from build123d import *

# Parameters (mm, degrees)
BOSS_EXTRU_1_DEPTH      = 320
ENL_V_MAT_EXTRU_1_DEPTH = 70
ESQUISSE3_R             = 150
BOSS_EXTRU_2_DEPTH      = 10
ESQUISSE4_R             = 1
ENL_V_MAT_EXTRU_2_DEPTH = 10


with BuildPart() as part:
    # Esquisse1 → Boss.-Extru.1 (new body)
    with BuildSketch(Plane(origin=(0, 0, 0), x_dir=(1, 0, 0), z_dir=(0, 1, 0))):
        with BuildLine():
            ThreePointArc((56.049273334, -8.002390035), (31.049273334, 16.997609965), (6.049273334, -8.002390035))
            Line((6.049273334, -8.002390035), (56.049273334, -8.002390035))
        make_face()
        with BuildLine():
            Line((56.049273334, -8.002390035), (6.049273334, -8.002390035))
            ThreePointArc((6.049273334, -8.002390035), (31.049273334, -33.002390035), (56.049273334, -8.002390035))
        make_face()
    extrude(amount=BOSS_EXTRU_1_DEPTH)

    # Esquisse2 → Enlèv. mat.-Extru.1 (cut)
    with BuildSketch(Plane(origin=(0, 0, 0), x_dir=(-1, 0, 0), z_dir=(0, -1, 0))):
        with BuildLine():
            Line((-31.049273334, -33.002390035), (-31.049273334, 16.997609965))
            ThreePointArc((-31.049273334, 16.997609965), (-56.049273334, -8.002390035), (-31.049273334, -33.002390035))
        make_face()
    extrude(amount=-ENL_V_MAT_EXTRU_1_DEPTH, mode=Mode.SUBTRACT)

    # Esquisse3 → Boss.-Extru.2 (add)
    with BuildSketch(Plane(origin=(0, 320, 0), x_dir=(1, 0, 0), z_dir=(0, 1, 0))):
        with Locations(Location((31.049273334, -8.002390035, 0), (0, 0, 270))):
            Circle(ESQUISSE3_R)
    extrude(amount=BOSS_EXTRU_2_DEPTH)

    # Esquisse4 → Enlèv. mat.-Extru.2 (cut)
    with BuildSketch(Plane(origin=(0, 330, 0), x_dir=(1, 0, 0), z_dir=(0, 1, 0))):
        with Locations(Location((-72.87377512, -68.002390035, 0), (0, 0, 270))):
            Circle(ESQUISSE4_R)
        with Locations(Location((-72.87377512, 51.997609965, 0), (0, 0, 270))):
            Circle(ESQUISSE4_R)
        with Locations(Location((31.049273334, 111.997609965, 0), (0, 0, 270))):
            Circle(ESQUISSE4_R)
        with Locations(Location((134.972321788, 51.997609965, 0), (0, 0, 270))):
            Circle(ESQUISSE4_R)
        with Locations(Location((134.972321788, -68.002390035, 0), (0, 0, 270))):
            Circle(ESQUISSE4_R)
        with Locations(Location((31.049273334, -128.002390035, 0), (0, 0, 270))):
            Circle(ESQUISSE4_R)
    extrude(amount=-ENL_V_MAT_EXTRU_2_DEPTH, mode=Mode.SUBTRACT)


solid = part.part
The model under review builds one solid part; all positions refer to its coordinate system, in mm. A direction names the side the tool comes from. Coordinates: 2 decimals unless noted, no trailing zeros. Loops run counter-clockwise (first coordinate to the right, second up) from the corner with the lowest first, then second, coordinate; pieces in that order, holes last. Notation, with made-up numbers: (11, 73) -> (47, 73) arc R21 cw to (47, 82) -> close; hole circle Ø7 at (69.25, 75). An arc over 180 degrees is marked (long way). Use a Markdown table: item, result. Add a question column.
1. Add section B-B on x = 40. Write out the cut boundary in (y, z).
2. Add section C-C on y = 90. Write out the cut boundary in (x, z).
3. To check wall thickness, follow line 1 (Y direction, x = -10, z = 107.5); line 2 (Z direction, x = 29.5, y = 308); line 3 (Z direction, x = 42, y = 220). State the ranges of each line that lie inside material, in increasing order.
4. Machinability: for faces 1 (the face through (33, 330, 6)), 2 (the face through (7.956, 157.76, -1.573)), 3 (the face through (31.049, 35, 8)), which of the approach directions +Z, -Z, +X, -X, +Y, -Y give a long, thin tool a straight path to every point of the face, cutting with its end or side? Answer none if there is none.
5. Add section D-D on x = -49. Write out the cut boundary in (y, z), plus the area to 3 significant figures.
6. Add section A-A on z = 18. Write out the cut boundary in (x, y).
7. Clearance check with flat-ended pins moving along their axes: pin 1 Ø3 at (y, z) = (57, 9) entering from +X; pin 2 Ø2.5 at (x, z) = (-72.87, 68) entering from +Y; pin 3 Ø12 at (x, y) = (26, 237.5) entering from -Z; pin 4 Ø3 at (x, z) = (134.97, -52) entering from -Y. State where each tip first meets the part, or that it passes through.
Returned:
| question | item | result |
|---|---|---|
| 1 | outline | (70, -15.34) -> (320, -15.34) -> (320, -141.73) -> (330, -141.73) -> (330, 157.74) -> (320, 157.74) -> (320, 31.35) -> (70, 31.35) -> close |
| 2 | outline | circle Ø50 at (31.05, 8) |
| 3 | line 1 | y = 320 to 330 |
| 3 | line 2 | z = -16.95 to 32.95 |
| 3 | line 3 | z = -14.47 to 30.48 |
| 4 | face 1 | +Z, -Z, +X, -X, +Y |
| 4 | face 2 | -Y |
| 4 | face 3 | +Z, -Z, +X, -Y |
| 5 | outline | (320, -118.85) -> (330, -118.85) -> (330, 134.86) -> (320, 134.86) -> close |
| 5 | area | 2,540 mm² |
| 6 | outline | (-118.62, 320) -> (8.14, 320) -> (8.14, 0) -> (31.05, 0) -> (31.05, 70) -> (53.96, 70) -> (53.96, 320) -> (180.72, 320) -> (180.72, 330) -> (-118.62, 330) -> close |
| 7 | pin 1 | stops at x = 31.05 |
| 7 | pin 2 | stops at y = 330 |
| 7 | pin 3 | stops at z = -17 |
| 7 | pin 4 | stops at y = 320 |
